Source: three-view drawing plus pictorial views. Frame: mm from the lowest corner of the part. A direction names the side the tool comes from. Coordinates: 2 decimals unless noted, no trailing zeros. Write each loop counter-clockwise with the first axis right and the second up, starting at its lowest first coordinate (ties: lowest second). Pieces come first, ordered by that corner, then holes. Notation, with made-up numbers: (58.25, 19.5) -> (68.25, 19.5) arc R25 ccw to (68.25, 43.5) -> close; hole circle Ø10 at (-9, -5.75). An arc over 180 degrees is marked (long way). One line per item, written item: value.
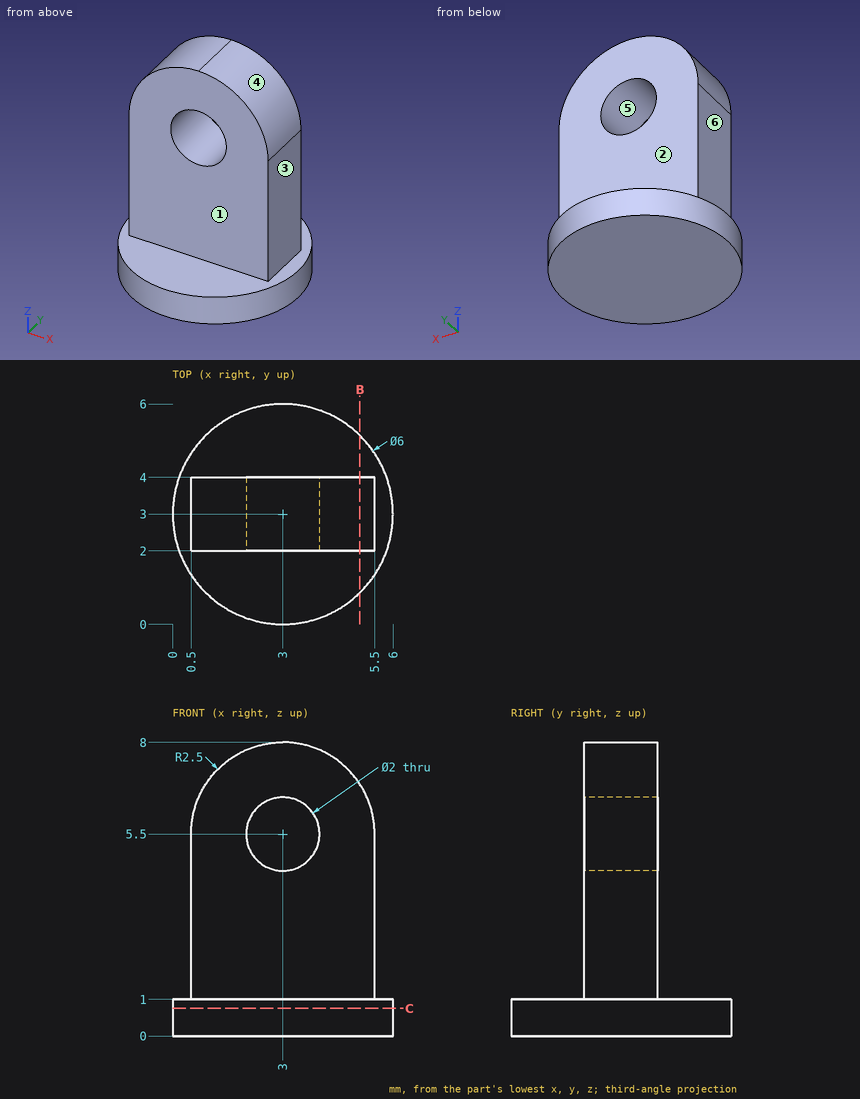
(1) Section C-C (z = 0.75). Return the cut outline in (x, y), then the cut area to 3 significant figures.
Responses:
outline: circle Ø6 at (3, 3)
area: 28.3 mm2
(2) Line query: line 1 (Z direction, x = 3, y = 2.6); line 2 (Y direction, x = 5.35, z = 1.25); line 3 (Z direction, x = 5.7, y = 3.55). Output: solid intervals per line, ascending. Write a range as [from, to].
Responses:
line 1: z = [0, 4.5], [6.5, 8]
line 2: y = [2, 4]
line 3: z = [0, 1]
(3) Pull-direction query (Z, two-part tool) for the marked faces 4, 5 and 6; classes: released by +Z, released by -Z, zero draft, split by the parting line, or undercut.
Responses:
face 4: released by +Z
face 5: undercut
face 6: zero draft
(4) First-contact query: pin 1 (2 mm diameter, centred on x = 5, z = 3.5, fed in from +Y); pin 2 (1.6 mm diameter, centred on y = 3.5, z = 3, fed in from -X); pin 3 (1 mm diameter, centred on y = 2.5, z = 3, fed in from +X). Flat tips, straight axial feed; report the tip coordinate or a pass-through.
Responses:
pin 1: stops at y = 4
pin 2: stops at x = 0.5
pin 3: stops at x = 5.5
(5) Section B-B (x = 5.1). Return the cut outline in (y, z), then the cut area to 3 significant figures.
Responses:
outline: (0.86, 0) -> (5.14, 0) -> (5.14, 1) -> (4, 1) -> (4, 6.86) -> (2, 6.86) -> (2, 1) -> (0.86, 1) -> close
area: 16.0 mm2
(6) Reachability of the marked faces 1, 2 and 3 from +Z, -Z, +X, -X, +Y, -Y: full face, straight path, thin tool, end or side. Return the list, or none.
Responses:
face 1: +Z, +X, -X, -Y
face 2: +Z, +X, -X, +Y
face 3: +Z, +X, +Y, -Y
